Source: CAD feature listing. Evaluate the final solid. Frame: model axes, mm. A direction names the side the tool comes from. Give positions to 0.01 mm unless a question says otherwise; leave off trailing zeros. Order: outer loops, then holes, each group sorted by start corner. A loop starts at its lowest first (then second) coordinate and runs counter-clockwise, first axis right, second up. Notation, with made-up numbers: (33, 3.5) -> (57, 3.5) arc R8 ccw to (57, 9.5) -> close; hole circle Ø3 at (72.5, -35). An arc over 180 degrees is marked (long way). Use CSV: the item, a comma, the result in double quotes.
```python
from build123d import *

# Parameters (mm, degrees)
F1_DEPTH = 1.27


with BuildPart() as f1:
    # F0 (on Front) → F1 (new body, symmetric)
    with BuildSketch(Plane.XZ):
        Polygon((-32.148205, 0), (0, 0), (32.198641, 0), (0, 43.575902), align=None)
        Polygon((24.49552, 3.727856), (-25.514841, 3.727856), (-2.913308, 34.21729), (-2.913308, 11.470481), (2.866663, 11.597541), (2.866663, 34.119293), align=None, mode=Mode.SUBTRACT)
    extrude(amount=F1_DEPTH, both=True)


solid = f1.part
```
1. Section query A-A on x = -9.5. Return loops of the section in (y, z).
Answer below:
outline,"(-1.27, 0) -> (1.27, 0) -> (1.27, 3.73) -> (-1.27, 3.73) -> close; (-1.27, 25.33) -> (1.27, 25.33) -> (1.27, 30.7) -> (-1.27, 30.7) -> close"
2. Access query for faces 5 (the flat face through (0, -1.27, 15)), 6 (the flat face through (0, 0, 3.728)). Directions: +Z, -Z, +X, -X, +Y, -Y. A direction counts if a zero-diameter tool reaches every point of the face in a straight line with its end or side. Return the directions, or none.
Answer below:
face 5,"+Z, -Z, +X, -X, -Y"
face 6,"+Y, -Y"
3. Pin query (flat end, axial travel): P1, Ø6, axis at x = -5, z = 23.5, coming from the -Y side; P2, Ø0.8, axis at x = -4, y = -0.5, coming from the +Z side. Return the tip coordinate at first contact, or that it passes through.
Answer below:
P1,"stops at y = -1.27"
P2,"stops at z = 38.7"
4. Section query C-C on z = 26. Return loops of the section in (x, y), plus the area to 3 significant figures.
Answer below:
outline,"(-12.97, -1.27) -> (-9, -1.27) -> (-9, 1.27) -> (-12.97, 1.27) -> close; (-2.91, -1.27) -> (2.87, -1.27) -> (2.87, 1.27) -> (-2.91, 1.27) -> close; (8.64, -1.27) -> (12.99, -1.27) -> (12.99, 1.27) -> (8.64, 1.27) -> close"
area,"35.8 mm²"
5. Mould query, pull axis X, two halves, no side actions, for faces 1 (the flat face through (0, 1.27, 15)), 2 (the flat face through (16.325, -0.018, 21.483)), 3 (the flat face through (-14.37, -0.02, 18.76)), 4 (the flat face through (-2.913, 0, 23)). Classes: released by +X, released by -X, zero draft, split by the parting line, or undercut.
Answer below:
face 1,"zero draft"
face 2,"released by +X"
face 3,"undercut"
face 4,"undercut"
6. Ray query, line 1 along X through (y, z) = (0.2, 22.5); line 2 along X through (y, z) = (-0.4, 13); line 3 along Z through (x, y) = (-1, 0.3). Return the intervals inside material, ascending.
Answer below:
line 1,"x = -15.55 to -11.6, -2.91 to 2.87, 11.14 to 15.57"
line 2,"x = -22.56 to -18.64, -2.91 to 2.87, 17.9 to 22.59"
line 3,"z = 0 to 3.73, 11.51 to 42.22"
7. Section query B-B on y = 0.7. Return loops of the section in (x, z).
Answer below:
outline,"(-32.15, 0) -> (32.2, 0) -> (0, 43.58) -> close; hole (-25.51, 3.73) -> (24.5, 3.73) -> (2.87, 34.12) -> (2.87, 11.6) -> (-2.91, 11.47) -> (-2.91, 34.22) -> close"
8. Section query D-D on z = 10. Return loops of the section in (x, y).
Answer below:
outline,"(-24.77, -1.27) -> (-20.87, -1.27) -> (-20.87, 1.27) -> (-24.77, 1.27) -> close; (20.03, -1.27) -> (24.81, -1.27) -> (24.81, 1.27) -> (20.03, 1.27) -> close"
